```python
from build123d import *

# Parameters (mm, degrees)
SKETCH1_W           = 130
SKETCH1_H           = 120
BOSS_EXTRUDE1_DEPTH = 3
CUT_EXTRUDE1_START  = -4
SKETCH2_R           = 6
CUT_EXTRUDE1_DEPTH  = 5


with BuildPart() as part:
    # Sketch1 → Boss-Extrude1 (new body)
    with BuildSketch(Plane(origin=(0, 0, 0), x_dir=(1, 0, 0), z_dir=(0, 1, 0))):
        Rectangle(SKETCH1_W, SKETCH1_H)
    extrude(amount=BOSS_EXTRUDE1_DEPTH)

    # Sketch2 → Cut-Extrude1 (cut)
    with BuildSketch(Plane(origin=(0, 3, 0), x_dir=(1, 0, 0), z_dir=(0, 1, 0)).offset(CUT_EXTRUDE1_START)):
        with Locations((44.5, 0)):
            Circle(SKETCH2_R)
    cut_extrude1 = extrude(amount=CUT_EXTRUDE1_DEPTH, mode=Mode.SUBTRACT)

    # Mirror1: Cut-Extrude1 across plane
    add(cut_extrude1.mirror(Plane(origin=(0, 0, 0), x_dir=(0, 0, 1), z_dir=(1, 0, 0))), mode=Mode.SUBTRACT)


solid = part.part
```
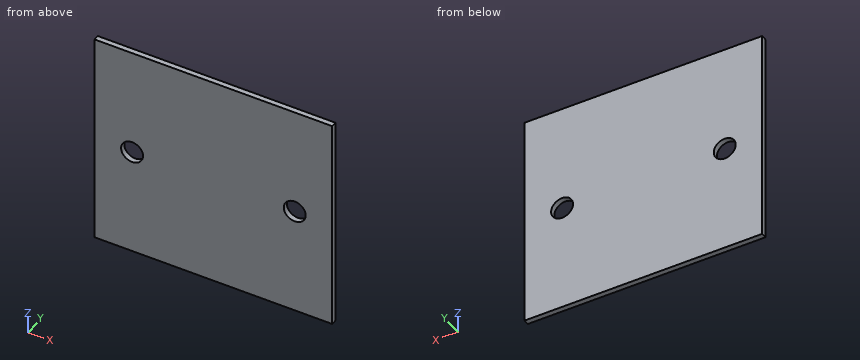
Here's how the part is built. I have some questions about the finished solid (model axes, mm). Coordinates: 2 decimals unless noted, no trailing zeros. Order: outer loops, then holes, each group sorted by start corner. A loop starts at its lowest first (then second) coordinate and runs counter-clockwise, first axis right, second up.
Item 1: I need wall thicknesses on probe 1 along X at (y, z) = (1.55, -0.5); probe 2 along Z at (x, y) = (44.5, 2.3); probe 3 along Z at (x, y) = (-47, 0.75). Which ranges of each line are inside material? Lowest first, please.
Response values:
probe 1: x = -65 to -50.48, -38.52 to 38.52, 50.48 to 65
probe 2: z = -60 to -6, 6 to 60
probe 3: z = -60 to -5.45, 5.45 to 60
Item 2: If we section it at A-A, the plane x = -44.5: List the corners of the cut face in (y, z) for me, then the cut area to 3 significant figures.
Response values:
outline: (0, -60) - (3, -60) - (3, -6) - (0, -6) - close; (0, 6) - (3, 6) - (3, 60) - (0, 60) - close
area: 324 mm2
Item 3: If we section it at B-B, the plane z = 0: List the corners of the cut face in (x, y) for me, then the cut area to 3 significant figures.
Response values:
outline: (-65, 0) - (-50.5, 0) - (-50.5, 3) - (-65, 3) - close; (-38.5, 0) - (38.5, 0) - (38.5, 3) - (-38.5, 3) - close; (50.5, 0) - (65, 0) - (65, 3) - (50.5, 3) - close
area: 318 mm2
Item 4: I'm going to push a flat-ended pin straight in: pin 1 Ø11 at (x, z) = (44.5, 0) entering from -Y. Where does the tip first touch, or does it pass through?
Response values:
pin 1: passes through
Item 5: If we section it at C-C, the plane x = 46.5: List the corners of the cut face in (y, z) for me, then the cut area to 3 significant figures.
Response values:
outline: (0, -60) - (3, -60) - (3, -5.66) - (0, -5.66) - close; (0, 5.66) - (3, 5.66) - (3, 60) - (0, 60) - close
area: 326 mm2
